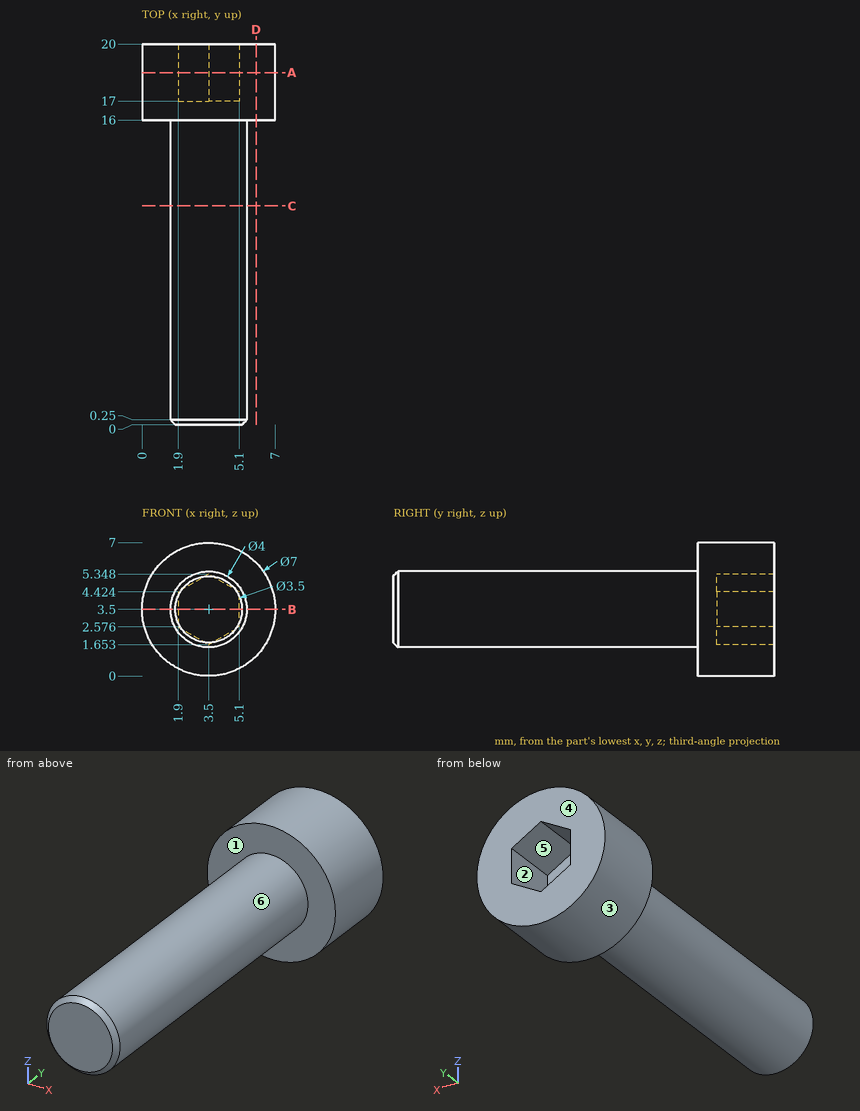
Design review of the part shown in the three views and the two pictorial views. Dimensions are in mm from the part's minimum x, y and z. A direction names the side the tool comes from. Coordinates: 2 decimals unless noted, no trailing zeros. Write each loop counter-clockwise with the first axis right and the second up, starting at its lowest first coordinate (ties: lowest second). Pieces come first, ordered by that corner, then holes.
(1) Add section D-D on x = 6. Give the boundary of the cut face in (y, z).
(2) Wall thickness on probe 1 along Y at (x, z) = (6, 1.75); probe 2 along Y at (x, z) = (3.75, 3.75); probe 3 along X at (y, z) = (8.75, 4) (1 decimal): over which ranges is each line inside the solid? List them lowest first.
(3) Add section C-C on y = 11.5. Give the boundary of the cut face in (x, z).
(4) The part is to be moulded in two halves that separate along Z. For the marked faces 1, 2 and 3, say which applies: +Z half, -Z half, draft (parallel to the pull), parting line (faces both ways), or undercut.
(5) Add section A-A on y = 18.5. Give the boundary of the cut face in (x, z), then the cut area to 3 significant figures.
(6) Add section B-B on z = 3.5. Give the boundary of the cut face in (x, y).
(7) Tool access review of the marked faces 4, 5 and 6: name each direction out of +Z, -Z, +X, -X, +Y, -Y from which nothing blocks a thin tool from reaching the whole face with its end or side.
(8) For pin 1 Ø1.5 at (y, z) = (8.5, 4.5) entering from -X (1 decimal); pin 2 Ø2 at (x, y) = (4.5, 6) entering from +Z, all flat-tipped, find the tip position at first contact; note any pin that passes through.
Answer sheet:
1. outline: (16, 1.05) - (20, 1.05) - (20, 5.95) - (16, 5.95) - close
2. probe 1: y = 16 to 20
2. probe 2: y = 0 to 17
2. probe 3: x = 1.6 to 5.4
3. outline: circle Ø4 at (3.5, 3.5)
4. face 1: draft
4. face 2: undercut
4. face 3: parting line
5. outline: circle Ø7 at (3.5, 3.5); hole (1.9, 2.58) - (3.5, 1.65) - (5.1, 2.58) - (5.1, 4.42) - (3.5, 5.35) - (1.9, 4.42) - close
5. area: 29.6 mm2
6. outline: (0, 16) - (1.5, 16) - (1.5, 0.25) - (1.75, 0) - (5.25, 0) - (5.5, 0.25) - (5.5, 16) - (7, 16) - (7, 20) - (5.1, 20) - (5.1, 17) - (1.9, 17) - (1.9, 20) - (0, 20) - close
7. face 4: +Z, -Z, +X, -X, +Y
7. face 5: +Y
7. face 6: -Y
8. pin 1: stops at x = 1.5
8. pin 2: stops at z = 5.5
